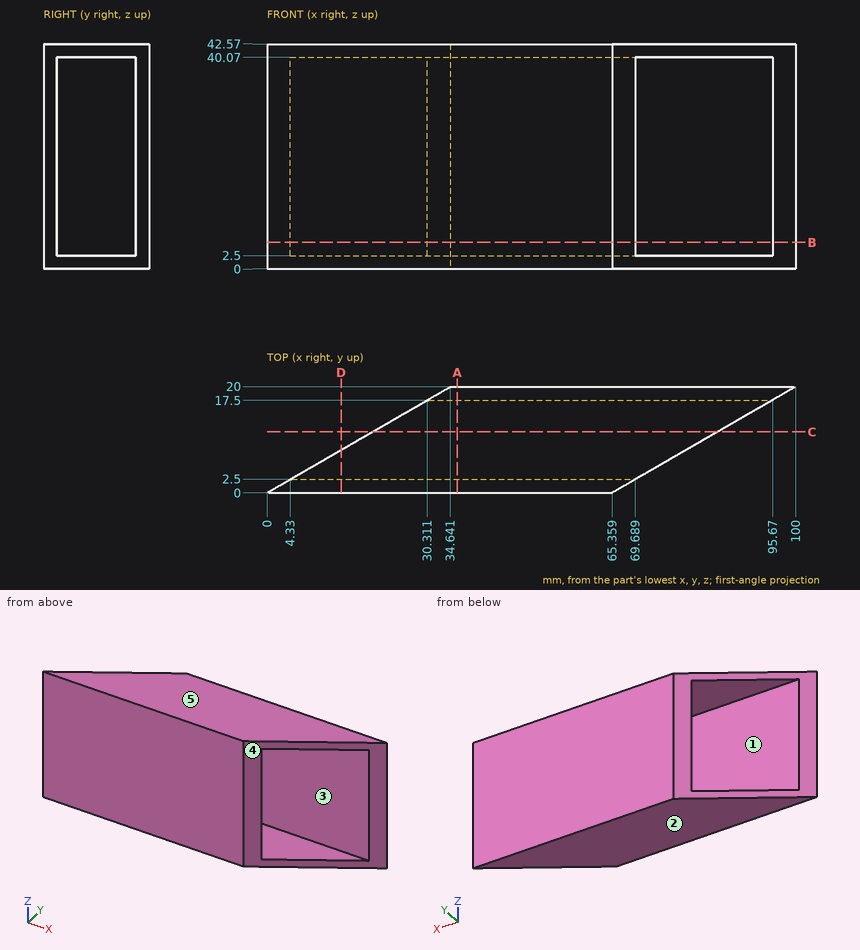
Answer from the drawing. Dimensions are ordinates in mm from the lowest x, y and z of the part. A direction names the side the tool comes from. Round coordinates to 2 decimals unless told otherwise and drop trailing zeros. Order: outer loops, then holes, each group sorted by start corner. A loop starts at its lowest first (then second) coordinate and runs counter-clockwise, first axis right, second up.
1) The part is cut by section B-B on z = 5. Write down the section's boundary in (x, y).
2) The part is cut by section D-D on x = 14. Write down the section's boundary in (y, z).
3) The part is cut by section A-A on x = 36. Write down the section's boundary in (y, z).
4) Flat-ended cylindrical pins translate along their axes: pin 1 (2 mm diameter, centred on x = 87, z = 37.5, fed in from -Y); pin 2 (4 mm diameter, centred on x = 32.5, z = 31.5, fed in from +Y); pin 3 (10 mm diameter, centred on y = 5.5, z = 7, fed in from -X); pin 4 (11.5 mm diameter, centred on x = 50, z = 15.5, fed in from -Y). Find the tip coordinate at first contact, or state that the pin passes through.
5) The mould has two halves that part along Z. Classify the marked faces 3, 4 and 5: released by +Z, released by -Z, zero draft, split by the parting line, or undercut.
6) For the marked faces 1 and 2, determine the directions among +Z, -Z, +X, -X, +Y, -Y from which every point of the face is accessible in a straight line to the end or side of a thin tool.
7) The part is cut by section C-C on y = 11.5. Write down the section's boundary in (x, z).
8) Straight lines are drawn through the part: L1, parallel to Z at x = 14, y = 4.25; L2, parallel to Y at x = 41, z = 30; L3, parallel to Y at x = 8, z = 23. For each, find the intervals that lie inside material, in ascending order.
Resolved:
1. outline: (0, 0) - (65.36, 0) - (69.69, 2.5) - (4.33, 2.5) - close; (30.31, 17.5) - (95.67, 17.5) - (100, 20) - (34.64, 20) - close
2. outline: (0, 0) - (8.08, 0) - (8.08, 2.5) - (2.5, 2.5) - (2.5, 40.07) - (8.08, 40.07) - (8.08, 42.57) - (0, 42.57) - close
3. outline: (0, 0) - (20, 0) - (20, 42.57) - (0, 42.57) - close; hole (2.5, 2.5) - (17.5, 2.5) - (17.5, 40.07) - (2.5, 40.07) - close
4. pin 1: stops at y = 17.5
4. pin 2: stops at y = 19.92
4. pin 3: stops at x = 0.87
4. pin 4: stops at y = 0
5. face 3: undercut
5. face 4: zero draft
5. face 5: released by +Z
6. face 1: +X, -X
6. face 2: -Z, +X, -X, +Y, -Y
7. outline: (19.92, 0) - (85.28, 0) - (85.28, 2.5) - (19.92, 2.5) - close; (19.92, 40.07) - (85.28, 40.07) - (85.28, 42.57) - (19.92, 42.57) - close
8. L1: z = 0 to 2.5, 40.07 to 42.57
8. L2: y = 0 to 2.5, 17.5 to 20
8. L3: y = 0 to 2.5
